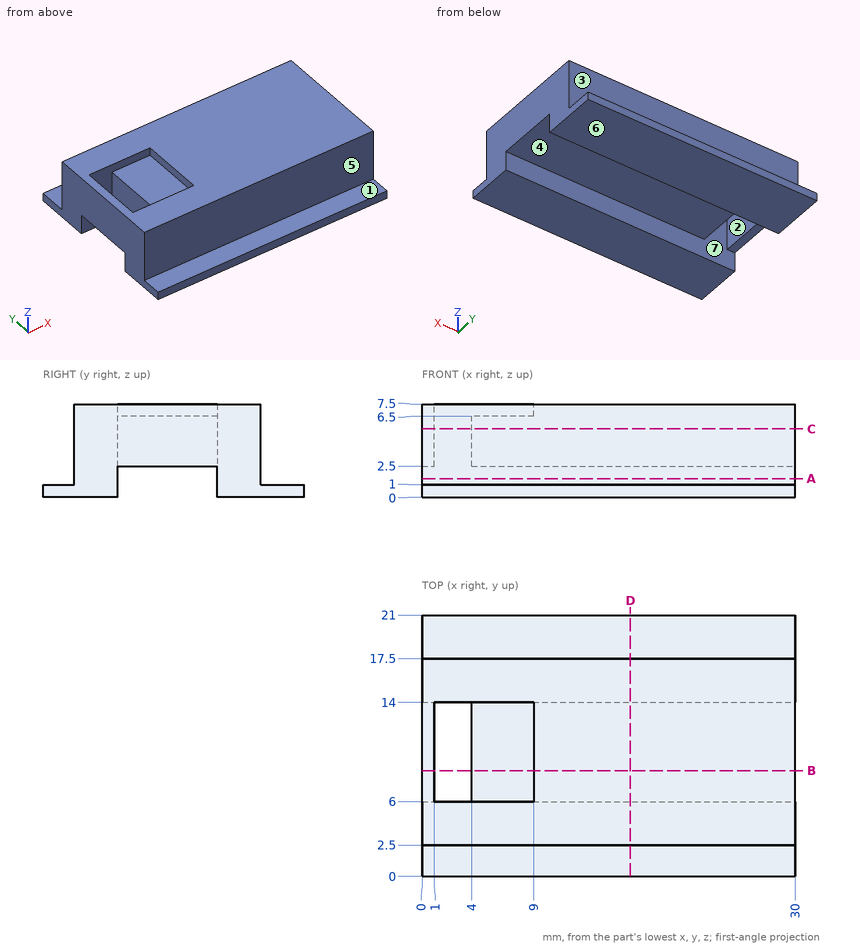
Print and shaded views of the part. All mm, measured from the part's lowest x, y and z. A direction names the side the tool comes from. Coordinates: 2 decimals unless noted, no trailing zeros. Write each loop counter-clockwise with the first axis right and the second up, starting at its lowest first coordinate (ties: lowest second). Pieces come first, ordered by that corner, then holes. Notation, with made-up numbers: (-22, 12) - (20, 12) arc R28 cw to (20, 41) - close; hole circle Ø7 at (-7.5, 26.25). An arc over 180 degrees is marked (long way). One line per question, with ' | ' between items. Start each with the question number.
Q1. Drill centre lines: line 1 (X direction, y = 10.5, z = 5); line 2 (Y direction, x = 12.25, z = 0.75); line 3 (Y direction, x = 20.5, z = 3). Where is each one in solid material? Low to high. Write a range as [from, to].
Q2. Pin check, flat tips, straight feed: pin 1 (2 mm diameter, centred on x = 15.5, z = 4.5, fed in from -Y); pin 2 (0.8 mm diameter, centred on x = 11.5, y = 2, fed in from +Z); pin 3 (0.5 mm diameter, centred on x = 0.5, y = 9.5, fed in from -Z). Stop position of each tip, or through.
Q3. Cut at A-A, the plane z = 1.5. List the corners of the cut face in (x, y), then the cut area to 3 significant figures.
Q4. 3-axis set-ups, long thin cutter, end or side, ignore diameter. For the marked faces 1, 2 and 3: which of +Z, -Z, +X, -X, +Y, -Y reach the whole face in a straight line?
Q5. Pull direction Y, two halves, no side cores. Call the marked faces 4, 5, 6 and 7: pulls with the +Y half, pulls with the -Y half, needs draft (parallel to the pull), parting line crosses it, or undercut.
Q6. Cut at B-B, the plane y = 8.5. List the corners of the cut face in (x, z), then the cut area to 3 significant figures.
Q7. Cut at C-C, the plane z = 5.5. List the corners of the cut face in (x, y), then the cut area to 3 significant figures.
Q8. Cut at D-D, the plane x = 16.75. List the corners of the cut face in (y, z), then the cut area to 3 significant figures.
Answer below:
1) line 1: [0, 1], [4, 30] | line 2: [0, 6], [14, 21] | line 3: [2.5, 17.5]
2) pin 1: y = 2.5 | pin 2: z = 1 | pin 3: z = 2.5
3) outline: (0, 2.5) - (30, 2.5) - (30, 6) - (0, 6) - close; (0, 14) - (30, 14) - (30, 17.5) - (0, 17.5) - close | area: 210 mm^2
4) face 1: +Z, +X, -X, -Y | face 2: +Z, -Z | face 3: +Z, +X, -X, +Y
5) face 4: undercut | face 5: pulls with the -Y half | face 6: needs draft | face 7: undercut
6) outline: (0, 2.5) - (1, 2.5) - (1, 7.5) - (0, 7.5) - close; (4, 2.5) - (30, 2.5) - (30, 7.5) - (9, 7.5) - (9, 6.5) - (4, 6.5) - close | area: 130 mm^2
7) outline: (0, 2.5) - (30, 2.5) - (30, 17.5) - (0, 17.5) - close; hole (1, 6) - (4, 6) - (4, 14) - (1, 14) - close | area: 426 mm^2
8) outline: (0, 0) - (6, 0) - (6, 2.5) - (14, 2.5) - (14, 0) - (21, 0) - (21, 1) - (17.5, 1) - (17.5, 7.5) - (2.5, 7.5) - (2.5, 1) - (0, 1) - close | area: 98.5 mm^2
